Could you check a few things on this model? Use its own coordinates, in mm. Face numbers are marked on the shaded views. Give positions to 0.01 mm unless a question says otherwise; leave off trailing zeros. Loops run counter-clockwise (first coordinate to the right, second up) from the corner with the lowest first, then second, coordinate; pieces in that order, holes last. Notation, with made-up numbers: (-8, 63) -> (30, 63) arc R17 ccw to (30, 96) -> close; hole circle Ø1 at (-8, -6.75). An arc over 180 degrees is marked (long way). Write item = value, one per line. Start each with the question number.
1) I want a section at B-B (y = -8). List the corners of the cut face in (x, z) for me.
2) I'm going to push flat-ended pins straight in: pin 1 Ø2 at (x, y) = (-3.5, -22.5) entering from +Z; pin 2 Ø1.5 at (x, y) = (1.5, -9.5) entering from -Z; pin 3 Ø1 at (x, y) = (3.5, -8.5) entering from +Z. Where does each tip first touch, or does it pass through?
3) If we mould it in two halves opening along X, with no side actions, what happens to the marked faces 1 and 2? For each: +X half, -X half, draft (parallel to the pull), parting line (faces both ways), or undercut.
4) I need wall thicknesses on probe 1 along Z at (x, y) = (0.5, -19); probe 2 along X at (y, z) = (-21, 4); probe 3 along X at (y, z) = (-17, 4). Which ranges of each line are inside material? Lowest first, please. Write a range as from..to.
5) I want a section at A-A (y = -23). List the corners of the cut face in (x, z) for me, and give its area (3 significant figures).
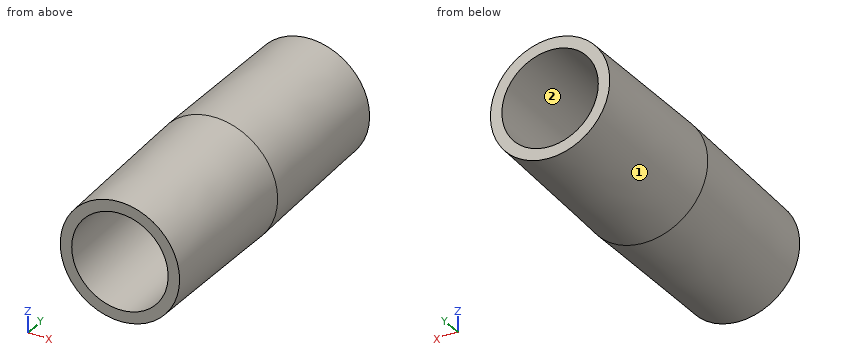
from build123d import *

# Parameters (mm, degrees)
F0_R     = 5.9817
F2_R     = 6.2865
F5_R     = 4.830776
F6_DEPTH = 50.8


with BuildPart() as f3:
    # F0 (on Front) → F3 section 0
    with BuildSketch(Plane.XZ):
        Circle(F0_R)
    # F2 (on offset) → F3 section 1
    with BuildSketch(Plane.XZ.offset(16.002)):
        Circle(F2_R)
    loft()

    # F4: F3 across plane


with BuildPart() as f3_1:
    add(f3.part)
    add(f3.part.mirror(Plane.XZ.offset(16.002)))

    # F5 (on face) → F6 (cut)
    with BuildSketch(Plane(origin=(0, 0, 0), x_dir=(-1, 0, 0), z_dir=(0, 1, 0))):
        Circle(F5_R)
    extrude(amount=-F6_DEPTH, mode=Mode.SUBTRACT)


solid = f3_1.part
Answer list:
q1.outline = circle Ø12.27 at (0, 0); hole circle Ø9.66 at (0, 0)
q2.pin_1 = 5.63
q2.pin_2 = -6.12
q2.pin_3 = 5.36
q3.face_1 = parting line
q3.face_2 = undercut
q4.probe_1 = -6.21..-4.8, 4.8..6.21
q4.probe_2 = -4.73..-2.71, 2.71..4.73
q4.probe_3 = -4.83..-2.71, 2.71..4.83
q5.outline = circle Ø12.31 at (0, 0); hole circle Ø9.66 at (0, 0)
q5.area = 45.6 mm^2
